Design review of the part built by this model. Coordinates are the model's own, in mm. A direction names the side the tool comes from. Coordinates: 2 decimals unless noted, no trailing zeros. Loops run counter-clockwise (first coordinate to the right, second up) from the corner with the lowest first, then second, coordinate; pieces in that order, holes last. Notation, with made-up numbers: M 75.25,41.5 L 87.25,41.5 A11 ccw 87.25,53.5 Z; hole C 26,3.5 d9. An arc over 180 degrees is marked long. Answer as a JSON object with one key per item and string values. Group by question number.
1. Insertion check: pin 1 (1.5 mm diameter, centred on y = 21, z = 1.5, fed in from -X); pin 2 (4.5 mm diameter, centred on x = -56.5, z = -3.5, fed in from +Y); pin 3 (0.5 mm diameter, centred on x = 57.5, z = 8.5, fed in from -Y). Each pin has a flat end and moves straight along its axis. Give the tip position at first contact, or say it passes through.
2. Machinability: for faces 4 (the flat face through (-60, 6, -9.29)), 5 (the cylindrical face through (-0.846, 38.949, 11.476)), 6 (the cylindrical face through (-48.196, 31.289, 0.182)), 7 (the flat face through (56.8, 6, 3.2)), 8 (the flat face through (-52, 27, 0)), which of the approach directions +Z, -Z, +X, -X, +Y, -Y give a long, thin tool a straight path to every point of the face, cutting with its end or side? Answer none if there is none.
3. To check wall thickness, follow probe 1 along X at (y, z) = (9.75, 0); probe 2 along X at (y, z) = (2.3, 0); probe 3 along Z at (x, y) = (-60, 13). State the ranges of each line that lie inside material, in increasing order.
4. Consider section A-A (y = 3.5). State the section outline as (x, z) points, then the cut area to 3 significant figures.
5. Consider section D-D (y = 29.5). State the section outline as (x, z) points, then the cut area to 3 significant figures.
6. Draft analysis for pull direction X (two halves, no side actions). For faces 1 (the flat face through (65, 0, 0)), 2 (the flat face through (-65.26, 25.58, 10.76)), 3 (the flat face through (59.9, 5.5, -7.61)), state which applies: +X half, -X half, draft (parallel to the pull), parting line (faces both ways), or undercut.
7. Consider section B-B (y = 12.5). State the section outline as (x, z) points, then the cut area to 3 significant figures.
8. Consider section C-C (z = -11). State the section outline as (x, y) points.
from build123d import *

# Parameters (mm, degrees)
EXTRUDE_START            = 13
EXTRUDE_1_DEPTH          = 26
CUT_EXTRUDE_1_DEPTH      = 70
CUT_EXTRUDE_1_DEPTH_BACK = 70
CUT_EXTRUDE_START        = 15
SKETCH_5_W               = 18
SKETCH_5_H               = 16.9
CUT_EXTRUDE_2_DEPTH      = 25
CUT_EXTRUDE_START_2      = 52.5
SKETCH_7_W               = 1.68
SKETCH_7_H               = 11.25
CUT_EXTRUDE_3_DEPTH      = 15
CUT_EXTRUDE_START_3      = -67.5
SKETCH_7_2_W             = 1.68
SKETCH_7_2_H             = 11.25
CUT_EXTRUDE_4_DEPTH      = 15


with BuildPart() as part:
    # 草图3 → 凸台-拉伸1 (new body)
    with BuildSketch(Plane.XY.offset(EXTRUDE_START)):
        with BuildLine():
            Line((-70, 15), (-60.389021238, 36.453077594))
            ThreePointArc((-60.389021238, 36.453077594), (-58.175420496, 39.035795149), (-54.913401609, 40))
            Line((-54.913401609, 40), (54.913401609, 40))
            ThreePointArc((54.913401609, 40), (58.175420496, 39.035795149), (60.389021238, 36.453077594))
            Line((60.389021238, 36.453077594), (70, 15))
            Line((70, 15), (70, 0))
            Line((70, 0), (50, 0))
            Line((50, 0), (50, 27))
            ThreePointArc((50, 27), (48.242640687, 31.242640687), (44, 33))
            Line((44, 33), (-44, 33))
            ThreePointArc((-44, 33), (-48.242640687, 31.242640687), (-50, 27))
            Line((-50, 27), (-50, 0))
            Line((-50, 0), (-70, 0))
            Line((-70, 0), (-70, 15))
        make_face()
    extrude(amount=-EXTRUDE_1_DEPTH)

    # 草图4 → 切除-拉伸1 (cut, two sides: drawn at the far end of the back side and taken through both)
    with BuildSketch(Plane(origin=(0, 0, 0), x_dir=(0, 0, -1), z_dir=(1, 0, 0)).offset(-CUT_EXTRUDE_1_DEPTH_BACK)):
        with BuildLine():
            Line((13, 36.42), (13, 33))
            Line((13, 33), (14, 33))
            Line((14, 33), (14, 41))
            Line((14, 41), (0, 41))
            Line((0, 41), (0, 40))
            ThreePointArc((0, 40), (1.385720645, 39.745514819), (2.590597511, 39.01527092))
            ThreePointArc((2.590597511, 39.01527092), (5.473035012, 37.839069568), (8.455602061, 38.731364009))
            ThreePointArc((8.455602061, 38.731364009), (11.436576626, 38.969213419), (13, 36.42))
        make_face()
        with BuildLine():
            Line((-14, 33), (-13, 33))
            Line((-13, 33), (-13, 36.42))
            ThreePointArc((-13, 36.42), (-11.436576626, 38.969213419), (-8.455602061, 38.731364009))
            ThreePointArc((-8.455602061, 38.731364009), (-5.473035012, 37.839069568), (-2.590597511, 39.01527092))
            ThreePointArc((-2.590597511, 39.01527092), (-1.385720645, 39.745514819), (0, 40))
            Line((0, 40), (0, 41))
            Line((0, 41), (-14, 41))
            Line((-14, 41), (-14, 33))
        make_face()
    extrude(amount=CUT_EXTRUDE_1_DEPTH + CUT_EXTRUDE_1_DEPTH_BACK, mode=Mode.SUBTRACT)

    # 草图5 → 切除-拉伸2 (cut)
    with BuildSketch(Plane(origin=(0, 0, 0), x_dir=(1, 0, 0), z_dir=(0, 1, 0)).offset(CUT_EXTRUDE_START)):
        with Locations((-61, 0)):
            Rectangle(SKETCH_5_W, SKETCH_5_H)
        with Locations((61, 0)):
            Rectangle(SKETCH_5_W, SKETCH_5_H)
    extrude(amount=CUT_EXTRUDE_2_DEPTH, mode=Mode.SUBTRACT)

    # 草图6 → 切除-旋转1 (revolve, cut)
    with BuildSketch(Plane.XY, mode=Mode.PRIVATE) as cut_revolve_1_sk:
        Polygon((-64.25, 0), (-64.25, 6), (-67.5, 6), (-67.5, 15), (-60, 15), (-60, 0), align=None)
    cut_revolve_1 = revolve(cut_revolve_1_sk.sketch.rotate(Axis((-60, 0, 0), (0, 1, 0)), 270), axis=Axis((-60, 0, 0), (0, 1, 0)), mode=Mode.SUBTRACT)

    # 镜向1: 切除-旋转1 across plane
    add(cut_revolve_1.mirror(Plane(origin=(0, 0, 0), x_dir=(0, 0, 1), z_dir=(1, 0, 0))), mode=Mode.SUBTRACT)

    # 草图7 → 切除-拉伸3 (cut)
    with BuildSketch(Plane(origin=(0, 0, 0), x_dir=(0, 0, -1), z_dir=(1, 0, 0)).offset(CUT_EXTRUDE_START_2)):
        with Locations((8.45, 5.625)):
            Rectangle(SKETCH_7_W, SKETCH_7_H)
        with Locations((-8.45, 5.625)):
            Rectangle(SKETCH_7_W, SKETCH_7_H)
    extrude(amount=CUT_EXTRUDE_3_DEPTH, mode=Mode.SUBTRACT)

    # 草图7<2> → 切除-拉伸4 (cut)
    with BuildSketch(Plane(origin=(0, 0, 0), x_dir=(0, 0, -1), z_dir=(1, 0, 0)).offset(CUT_EXTRUDE_START_3)):
        with Locations((8.45, 5.625)):
            Rectangle(SKETCH_7_2_W, SKETCH_7_2_H)
        with Locations((-8.45, 5.625)):
            Rectangle(SKETCH_7_2_W, SKETCH_7_2_H)
    extrude(amount=CUT_EXTRUDE_4_DEPTH, mode=Mode.SUBTRACT)


solid = part.part
Findings below:
{
 "1": {"pin 1": "stops at x = -52", "pin 2": "stops at y = 6", "pin 3": "stops at y = 11.25"},
 "2": {"face 4": "-Y", "face 5": "+X, -X, +Y", "face 6": "+Z, -Z, -Y", "face 7": "+Y", "face 8": "-X, +Y"},
 "3": {"probe 1": "x = -70 to -67.5, -52.5 to -50, 50 to 52.5, 67.5 to 70", "probe 2": "x = -70 to -64.25, -55.75 to -50, 50 to 55.75, 64.25 to 70", "probe 3": "z = -13 to -7.5, 7.5 to 13"},
 "4": {"outline": "M -70,-13 L -50,-13 L -50,13 L -70,13 Z; M 50,-13 L 70,-13 L 70,13 L 50,13 Z; hole M -67.5,-9.29 L -52.5,-9.29 L -52.5,-7.61 L -67.5,-7.61 Z; hole M -67.5,7.61 L -52.5,7.61 L -52.5,9.29 L -67.5,9.29 Z; hole C -60,0 d8.5; hole M 52.5,-9.29 L 67.5,-9.29 L 67.5,-7.61 L 52.5,-7.61 Z; hole M 52.5,7.61 L 67.5,7.61 L 67.5,9.29 L 52.5,9.29 Z; hole C 60,0 d8.5", "area": "826 mm^2"},
 "5": {"outline": "M -63.5,-13 L -49.45,-13 L -49.45,13 L -63.5,13 L -63.5,8.45 L -52,8.45 L -52,-8.45 L -63.5,-8.45 Z; M 49.45,-13 L 63.5,-13 L 63.5,-8.45 L 52,-8.45 L 52,8.45 L 63.5,8.45 L 63.5,13 L 49.45,13 Z", "area": "342 mm^2"},
 "6": {"face 1": "draft", "face 2": "-X half", "face 3": "undercut"},
 "7": {"outline": "M -70,-13 L -50,-13 L -50,13 L -70,13 Z; M 50,-13 L 70,-13 L 70,13 L 50,13 Z; hole C -60,0 d15; hole C 60,0 d15", "area": "687 mm^2"},
 "8": {"outline": "M -70,0 L -50,0 L -50,27 A6 cw -44,33 L 44,33 A6 cw 50,27 L 50,0 L 70,0 L 70,15 L 60.39,36.45 A6 ccw 58,39.15 L -58,39.15 A6 ccw -60.39,36.45 L -70,15 Z"}
}
